Here's how the part is built. I have some questions about the finished solid (model axes, mm). A direction names the side the tool comes from. Round coordinates to 2 decimals unless told otherwise and drop trailing zeros. Write each loop counter-clockwise with the first axis right and the second up, starting at its lowest first coordinate (ties: lowest second). Pieces come first, ordered by that corner, then holes. Notation, with made-up numbers: (-6, 61.5) -> (12, 61.5) arc R7 ccw to (12, 67.5) -> close; hole circle Ø7 at (-28.5, -19). An arc over 180 degrees is marked (long way). Answer in a Markdown table with one row per item. Add a question column.
from build123d import *

# Parameters (mm, degrees)
SKETCH016_AS_DRAWN_R                 = 13.5
EXTRUDE001_DEPTH                     = 30
EXTRUDE001_ONTO_SKETCH016_ROLL_ANGLE = 90
SKETCH017_AS_DRAWN_W                 = 2
SKETCH017_AS_DRAWN_H                 = 25
EXTRUDE002_DEPTH                     = 20
EXTRUDE002_ONTO_SKETCH017_ROLL_ANGLE = 90
SKETCH020_W                          = 40
SKETCH020_H                          = 28
EXTRUDE003_DEPTH                     = 3
EXTRUDE004_DEPTH                     = 3
SKETCH021_R                          = 1.25
EXTRUDE005_DEPTH                     = 15
EXTRUDE006_DEPTH                     = 15
SKETCH023_W                          = 45
SKETCH023_H                          = 10
SKETCH_R                             = 1.5
EXTRUDE_DEPTH                        = 38
SKETCH014_W                          = 16
SKETCH014_H                          = 20
BOX_W                                = 34
BOX_H                                = 50
BOX_DEPTH                            = 70


with BuildPart() as extrude_tube_hole:
    # Sketch016 as drawn → Extrude001 (new)
    with BuildSketch(Plane.XY):
        with Locations((0, 50)):
            Circle(SKETCH016_AS_DRAWN_R)
    extrude(amount=-EXTRUDE001_DEPTH)


with BuildPart() as extrude_tube_hole_1:
    # Extrude001 onto Sketch016 roll: moved
    add(extrude_tube_hole.part.rotate(Axis((0, 0, 0), (1, 0, 0)), EXTRUDE001_ONTO_SKETCH016_ROLL_ANGLE))


with BuildPart() as extrude_tube_hole_2:
    # Extrude001 onto Sketch016 placement: moved
    add(extrude_tube_hole_1.part)


with BuildPart() as extrude_tube_hole_3:
    # Extrude001 placement: moved
    add(extrude_tube_hole_2.part.moved(Location((0, -1, 0))))


with BuildPart() as arc_ext:
    # Sketch017 as drawn → Extrude002 (new)
    with BuildSketch(Plane.XY):
        Polygon((3.5, 35.5), (20, 41.505509), (20, 20), (3.5, 20), align=None)
        Polygon((-3.5, 35.5), (-20, 41.505509), (-20, 20), (-3.5, 20), align=None)
        with Locations((0, 27.5)):
            Rectangle(SKETCH017_AS_DRAWN_W, SKETCH017_AS_DRAWN_H)
    extrude(amount=-EXTRUDE002_DEPTH)


with BuildPart() as arc_ext_1:
    # Extrude002 onto Sketch017 roll: moved
    add(arc_ext.part.rotate(Axis((0, 0, 0), (1, 0, 0)), EXTRUDE002_ONTO_SKETCH017_ROLL_ANGLE))


with BuildPart() as arc_ext_2:
    # Extrude002 onto Sketch017 placement: moved
    add(arc_ext_1.part)


with BuildPart() as arc_ext_3:
    # Extrude002 placement: moved
    add(arc_ext_2.part.moved(Location((0, -1, 0))))


with BuildPart() as extrude003:
    # Sketch020 → Extrude003 (new body)
    with BuildSketch(Plane.XY):
        with Locations((0, 47)):
            Rectangle(SKETCH020_W, SKETCH020_H)
    extrude(amount=EXTRUDE003_DEPTH)


with BuildPart() as extrude003_1:
    # Extrude003 placement: moved
    add(extrude003.part.moved(Location((0, 0, 68))))


with BuildPart() as extrude004:
    # Sketch020 → Extrude004 (new body)
    with BuildSketch(Plane.XY):
        with Locations((0, 47)):
            Rectangle(SKETCH020_W, SKETCH020_H)
    extrude(amount=EXTRUDE004_DEPTH)


with BuildPart() as extrude004_1:
    # Extrude004 placement: moved
    add(extrude004.part.moved(Location((0, 0, 14))))


with BuildPart() as extrude005:
    # Sketch021 → Extrude005 (new body)
    with BuildSketch(Plane.XY):
        with Locations((-12.5, 45)):
            Circle(SKETCH021_R)
        with Locations((12.5, 45)):
            Circle(SKETCH021_R)
        with Locations((0, 37)):
            Circle(SKETCH021_R)
    extrude(amount=EXTRUDE005_DEPTH)


with BuildPart() as extrude005_1:
    # Extrude005 placement: moved
    add(extrude005.part.moved(Location((0, 0, 13))))


with BuildPart() as extrude006:
    # Sketch021 → Extrude006 (new body)
    with BuildSketch(Plane.XY):
        with Locations((-12.5, 45)):
            Circle(SKETCH021_R)
        with Locations((12.5, 45)):
            Circle(SKETCH021_R)
        with Locations((0, 37)):
            Circle(SKETCH021_R)
    extrude(amount=EXTRUDE006_DEPTH)


with BuildPart() as extrude006_1:
    # Extrude006 placement: moved
    add(extrude006.part.moved(Location((0, 0, 58))))


with BuildPart() as sweep002:
    # Sweep002: sweep along a path in Sketch022
    with BuildLine(Plane.XZ) as sweep002_path:
        ThreePointArc((-18, 17), (0, -1), (18, 17))
    # Sketch023 → Sweep002 (sweep)
    with BuildSketch(Plane.YZ):
        with Locations((21.5, -6)):
            Rectangle(SKETCH023_W, SKETCH023_H)
    sweep(path=sweep002_path.line)


with BuildPart() as fusion001:
    # Sketch → Extrude (new body)
    with BuildSketch(Plane.YZ):
        with Locations((7.25, 31.5)):
            Circle(SKETCH_R)
        with BuildLine():
            Line((61, 63), (32.5, 63))
            ThreePointArc((32.5, 63), (27.196699, 60.803301), (25, 55.5))
            Line((25, 55.5), (25, 28.5))
            ThreePointArc((25, 28.5), (27.196699, 23.196699), (32.5, 21))
            Line((32.5, 21), (61, 21))
            Line((61, 21), (61, 63))
        make_face()
        with BuildLine():
            Line((61, 15), (32.5, 15))
            ThreePointArc((32.5, 15), (27.196699, 12.803301), (25, 7.5))
            Line((25, 7.5), (25, -2))
            Line((25, -2), (61, -2))
            Line((61, -2), (61, 15))
        make_face()
        with BuildLine():
            Line((20, 47), (20, -2))
            Line((20, -2), (-0.5, -2))
            Line((-0.5, -2), (-0.5, 27))
            Line((-0.5, 27), (15, 27))
            Line((15, 27), (15, 47))
            ThreePointArc((20, 47), (17.5, 49.5), (15, 47))
        make_face()
    extrude(amount=EXTRUDE_DEPTH)


with BuildPart() as fusion001_1:
    # Extrude placement: moved
    add(fusion001.part.moved(Location((-19, 0, 0))))

    # Fusion001: union Extrude-tube-hole, arc-ext, Extrude003, Extrude004, Extrude005, Extrude006, Sweep002
    add(extrude_tube_hole_3.part)
    add(arc_ext_3.part)
    add(extrude003_1.part)
    add(extrude004_1.part)
    add(extrude005_1.part)
    add(extrude006_1.part)
    add(sweep002.part)


with BuildPart() as sweep_body:
    # Sweep: sweep along a path in Sketch015
    with BuildLine(Plane.XZ) as sweep_path:
        ThreePointArc((4, 40.834849), (0, 60), (-4, 40.834849))
    # Sketch014 → Sweep (sweep)
    with BuildSketch(Plane(origin=(0, -1, 0), x_dir=(0, 1, 0), z_dir=(1, 0, 0))):
        with Locations((8, 75)):
            Rectangle(SKETCH014_W, SKETCH014_H)
    sweep(path=sweep_path.line)


with BuildPart() as fusion:
    # Sweep001: sweep along a path in Sketch019
    with BuildLine(Plane.XZ) as sweep001_path:
        ThreePointArc((9.439809, 46.7), (0, 60), (-9.439809, 46.7))
    # Sketch018 → Sweep001 (sweep)
    with BuildSketch(Plane(origin=(0, -1, 0), x_dir=(0, 1, 0), z_dir=(1, 0, 0))):
        Polygon((16, 65), (16, 83.121211), (45, 83.121211), align=None)
    sweep(path=sweep001_path.line)

    # Fusion: union Sweep body
    add(sweep_body.part)


with BuildPart() as cut001:
    # Box → Box (new body)
    with BuildSketch(Plane(origin=(-17, 0, 0), x_dir=(1, 0, 0), z_dir=(0, 0, 1))):
        with Locations((17, 25)):
            Rectangle(BOX_W, BOX_H)
    extrude(amount=BOX_DEPTH)

    # Cut: cut Fusion
    add(fusion.part, mode=Mode.SUBTRACT)

    # Cut001: cut Fusion001
    add(fusion001_1.part, mode=Mode.SUBTRACT)


solid = cut001.part
Item 1: For P1, Ø2, axis at x = 2, y = 19.5, coming from the +Z side; P2, Ø13.5, axis at x = 0, y = 43, coming from the +Z side; P3, Ø1.6, axis at x = 6, z = 69.5, coming from the +Y side; P4, Ø2, axis at x = 12.5, y = 45, coming from the -Z side, each with a flat end and sliding along its axis, tell me the tip position at first contact or that it passes through.
Item 2: If we section it at C-C on z = 44: Please give me the cut outline in (x, y), then the cut area to 3 significant figures.
Item 3: If we section it at B-B on z = 31.5: Please give me the cut outline in (x, y).
Item 4: I need wall thicknesses on line 1 along X through (y, z) = (12.5, 29); line 2 along Z through (x, y) = (6.5, 40.5); line 3 along Y through (x, z) = (-2, 31.5). Which ranges of each line are inside material? Lowest first, please. Write a range as from..to.
Item 5: If we mould it in two halves opening along Z, with no side actions, what happens to faces 4 (the flat face through (-2, 7, 27)), 5 (the flat face through (0, 42, 68)), 6 (the flat face through (0, 20, 24)), 7 (the flat face through (0, 41, 21))? For each: pulls with the +Z half, pulls with the -Z half, needs draft (parallel to the pull), parting line crosses it, or undercut.
Item 6: On a 3-axis mill with a long thin cutter (end or side, diameter ignored), from which of +Z, -Z, +X, -X, +Y, -Y can I reach the whole of each face in a straight line? I mean faces 1 (the flat face through (0, 33, 16)), 2 (the flat face through (0, 41, 63)), 3 (the flat face through (4.8, 15, 36.2)). Say none if no direction works.
Item 7: If we section it at A-A on x = 0: Give the number of separate pieces and of enclosed holes in the cut face, then the cut area to 3 significant figures.
Results list:
| question | item | result |
|---|---|---|
| 1 | P1 | z = 68.34 |
| 1 | P2 | z = 68 |
| 1 | P3 | y = 33 |
| 1 | P4 | through |
| 2 | outline | (-17, 20) -> (-12.09, 20) -> (-12.09, 25) -> (-17, 25) -> close; (-13.75, 0) -> (-12.09, 0) -> (-12.09, 15) -> (-13.75, 15) -> close; (12.09, 0) -> (13.75, 0) -> (13.75, 15) -> (12.09, 15) -> close; (12.09, 20) -> (17, 20) -> (17, 25) -> (12.09, 25) -> close |
| 2 | area | 98.7 mm² |
| 3 | outline | (-17, 20) -> (17, 20) -> (17, 25) -> (-17, 25) -> close; (-3.5, 0) -> (-1, 0) -> (-1, 5.75) -> (-3.5, 5.75) -> close; (-3.5, 8.75) -> (-1, 8.75) -> (-1, 15) -> (-3.5, 15) -> close; (1, 0) -> (3.5, 0) -> (3.5, 5.75) -> (1, 5.75) -> close; (1, 8.75) -> (3.5, 8.75) -> (3.5, 15) -> (1, 15) -> close |
| 4 | line 1 | -3.5..-1, 1..3.5 |
| 4 | line 2 | 17..21, 63..68 |
| 4 | line 3 | 0..5.75, 8.75..15, 20..25 |
| 5 | face 4 | pulls with the -Z half |
| 5 | face 5 | pulls with the +Z half |
| 5 | face 6 | needs draft |
| 5 | face 7 | undercut |
| 6 | face 1 | -Z, +X, -X, +Y |
| 6 | face 2 | +X, -X, +Y |
| 6 | face 3 | -Z, +X, -X |
| 7 | separate pieces | 4 |
| 7 | enclosed holes | 0 |
| 7 | area | 508 mm² |
